Build history of the part. All positions in model axes, mm. Face numbers are marked on the shaded views. A direction names the side the tool comes from. Give positions to 0.01 mm unless a question says otherwise; leave off trailing zeros. Write each loop counter-clockwise with the first axis right and the second up, starting at its lowest first coordinate (ties: lowest second). Pieces come first, ordered by that corner, then holes. Notation, with made-up numbers: M 85.25,-19 L 94.25,-19 A15 cw 94.25,-9 Z; hole C 50,87 d1. An arc over 180 degrees is marked long. Return JSON: item names as keys, results as strings. Group by question number.
Q1. Flat gauge pins, fed straight in: pin 1 Ø2 at (y, z) = (1.5, -1.5) entering from -X; pin 2 Ø3 at (y, z) = (-57.5, 0.5) entering from +X; pin 3 Ø3 at (y, z) = (-67, 2.5) entering from -X. Where does each tip first touch, or does it go through?
Q2. Wall check: probe 1 along Y at (x, z) = (147, -0.5); probe 2 along X at (y, z) = (-65.5, 2); probe 3 along X at (y, z) = (-2.5, 2.25). Give the ranges that are in metal, low to high.
Q3. Tool access for the marked faces 1 and 2: list every direction of +Z, -Z, +X, -X, +Y, -Y with a clear straight run to the whole face (end or side of a thin tool).
Q4. Band-saw the part on A-A, the plane y = -46. Give the cut face in (x, z).
from build123d import *

# Parameters (mm, degrees)
WYCI_GNI_CIE_PO_CIE_CE1_PROFILE_R = 3.5
SZKIC26_R                         = 4
SZKIC26_R_2                       = 2.85
WYTNIJ_WYCI_GNI_CIE1_DEPTH        = 1.5
SZKIC36_R                         = 4
SZKIC36_R_2                       = 2.85
WYTNIJ_WYCI_GNI_CIE3_DEPTH        = 1.5
SZKIC46_R                         = 4
SZKIC46_R_2                       = 1.6
WYTNIJ_WYCI_GNI_CIE4_DEPTH        = 0.8
WYTNIJ_WYCI_GNI_CIE5_START        = 0.8
SZKIC53_R                         = 4
SZKIC53_R_2                       = 1.6
WYTNIJ_WYCI_GNI_CIE5_DEPTH        = 0.8


with BuildPart() as part:
    # Wyciągnięcie po ścieżce1: sweep along a path in Szkic1
    with BuildLine(Plane.XY) as wyci_gni_cie_po_cie_ce1_path:
        Line((183, 0), (10, 0))
        ThreePointArc((10, 0), (2.928932188, -2.928932188), (0, -10))
        Line((0, -10), (0, -110))
    # Wyciągnięcie po ścieżce1 profile (on start of the path) → Wyciągnięcie po ścieżce1 (sweep)
    with BuildSketch(Plane(origin=(183, 0, 0), x_dir=(0, 0, -1), z_dir=(-1, 0, 0))):
        Circle(WYCI_GNI_CIE_PO_CIE_CE1_PROFILE_R)
    sweep(path=wyci_gni_cie_po_cie_ce1_path.line)

    # Szkic26 → Wytnij-wyciągnięcie1 (cut)
    with BuildSketch(Plane(origin=(0, -105, 0), x_dir=(-1, 0, 0), z_dir=(0, -1, 0))):
        Circle(SZKIC26_R)
        with Locations(Location((0, 0, 0), (0, 0, 180))):
            Circle(SZKIC26_R_2, mode=Mode.SUBTRACT)
    extrude(amount=-WYTNIJ_WYCI_GNI_CIE1_DEPTH, mode=Mode.SUBTRACT)

    # Szkic36 → Wytnij-wyciągnięcie3 (cut)
    with BuildSketch(Plane(origin=(0, -85, 0), x_dir=(-1, 0, 0), z_dir=(0, -1, 0))):
        Circle(SZKIC36_R)
        with Locations(Location((0, 0, 0), (0, 0, 180))):
            Circle(SZKIC36_R_2, mode=Mode.SUBTRACT)
    extrude(amount=-WYTNIJ_WYCI_GNI_CIE3_DEPTH, mode=Mode.SUBTRACT)

    # Szkic46 → Wytnij-wyciągnięcie4 (cut)
    with BuildSketch(Plane(origin=(181.5, 0, 0), x_dir=(0, 0, -1), z_dir=(1, 0, 0))):
        Circle(SZKIC46_R)
        with Locations(Location((0, 0, 0), (0, 0, 90))):
            Circle(SZKIC46_R_2, mode=Mode.SUBTRACT)
    extrude(amount=-WYTNIJ_WYCI_GNI_CIE4_DEPTH, mode=Mode.SUBTRACT)

    # Szkic53 → Wytnij-wyciągnięcie5 (cut)
    with BuildSketch(Plane(origin=(119, 0, 0), x_dir=(0, 0, -1), z_dir=(1, 0, 0)).offset(WYTNIJ_WYCI_GNI_CIE5_START)):
        Circle(SZKIC53_R)
        with Locations(Location((0, 0, 0), (0, 0, 90))):
            Circle(SZKIC53_R_2, mode=Mode.SUBTRACT)
    extrude(amount=-WYTNIJ_WYCI_GNI_CIE5_DEPTH, mode=Mode.SUBTRACT)


solid = part.part
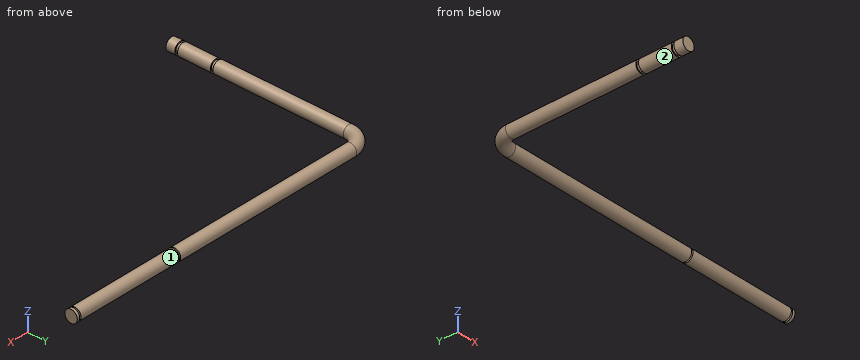
From the geometry:
{
 "1": {"pin 1": "stops at x = 1.91", "pin 2": "stops at x = 3.5", "pin 3": "stops at x = -3.35"},
 "2": {"probe 1": "y = -3.46 to 3.46", "probe 2": "x = -2.87 to 2.87", "probe 3": "x = -0.23 to 119, 119.8 to 180.7, 181.5 to 183"},
 "3": {"face 1": "+X", "face 2": "-Y"},
 "4": {"outline": "C 0,0 d7"}
}
